Check sheet for the drawn part. Datum: minimum x, y, z corner. Units: mm. A direction names the side the tool comes from. Round coordinates to 2 decimals unless told otherwise and drop trailing zeros. Write each loop counter-clockwise with the first axis right and the second up, starting at its lowest first coordinate (ties: lowest second). Pieces come first, ordered by that corner, then holes.
Item 1: Cross-section at D-D on x = 2.5. Enter the section's corners in (y, z).
Item 2: Release check for a two-part mould opening along Z. For the marked faces 3, 4 and 5 record: +Z half, -Z half, draft (parallel to the pull), parting line (faces both ways), or undercut.
Item 3: Cross-section at C-C on x = 17.25. Enter the section's corners in (y, z).
Item 4: Tool access check on the marked faces 1 and 2. Record the directions out of +Z, -Z, +X, -X, +Y, -Y that give a thin tool (end or side, any length) a straight path to the whole face; none if there is none.
Item 5: Material ranges on line 1 (X direction, y = 0.95, z = 2.9); line 2 (X direction, y = 1.2, z = 4.15); line 3 (Z direction, x = 14.5, y = 0.85), recorded low to high.
Item 6: Cross-section at B-B on y = 1.25. Enter the section's corners in (x, z).
Item 7: Cross-section at A-A on z = 3. Enter the section's corners in (x, y), plus the area to 3 significant figures.
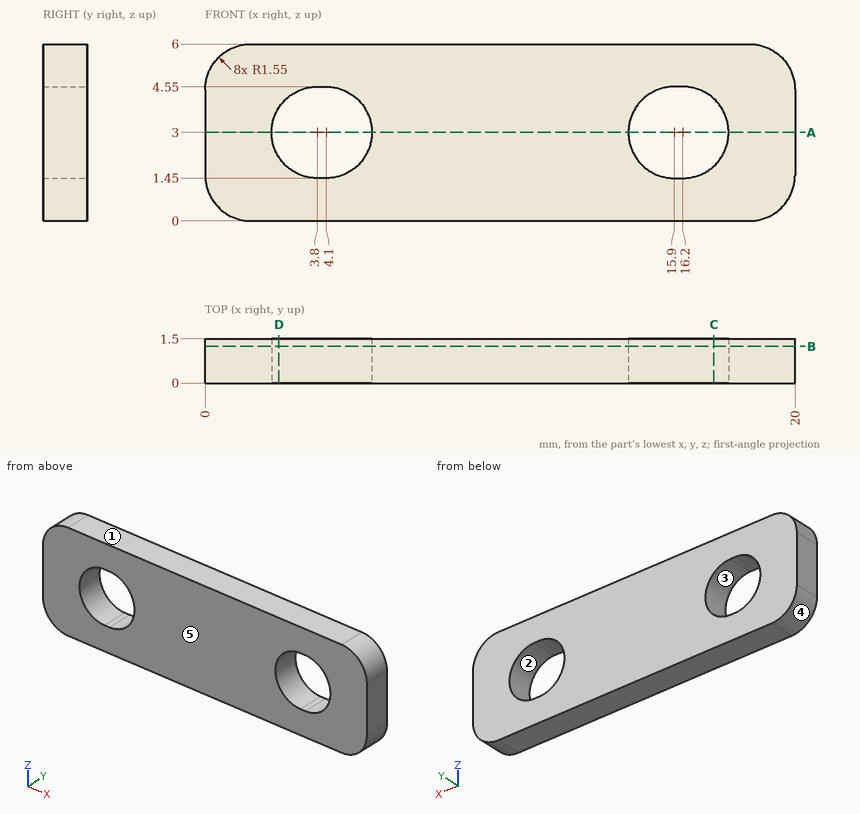
Response values:
1. outline: (0, 0) - (1.5, 0) - (1.5, 2.16) - (0, 2.16) - close; (0, 3.84) - (1.5, 3.84) - (1.5, 6) - (0, 6) - close
2. face 3: undercut
2. face 4: -Z half
2. face 5: draft
3. outline: (0, 0) - (1.5, 0) - (1.5, 1.86) - (0, 1.86) - close; (0, 4.14) - (1.5, 4.14) - (1.5, 6) - (0, 6) - close
4. face 1: +Z, +X, -X, +Y, -Y
4. face 2: +Y, -Y
5. line 1: x = 0 to 2.25, 5.65 to 14.35, 17.75 to 20
5. line 2: x = 0 to 2.76, 5.14 to 14.86, 17.24 to 20
5. line 3: z = 0 to 2.33, 3.67 to 6
6. outline: (0, 1.55) arc R1.55 ccw to (1.55, 0) - (18.45, 0) arc R1.55 ccw to (20, 1.55) - (20, 4.45) arc R1.55 ccw to (18.45, 6) - (1.55, 6) arc R1.55 ccw to (0, 4.45) - close; hole (3.8, 1.45) - (4.1, 1.45) arc R1.55 ccw to (4.1, 4.55) - (3.8, 4.55) arc R1.55 ccw to start; hole (15.9, 1.45) - (16.2, 1.45) arc R1.55 ccw to (16.2, 4.55) - (15.9, 4.55) arc R1.55 ccw to start
7. outline: (0, 0) - (2.25, 0) - (2.25, 1.5) - (0, 1.5) - close; (5.65, 0) - (14.35, 0) - (14.35, 1.5) - (5.65, 1.5) - close; (17.75, 0) - (20, 0) - (20, 1.5) - (17.75, 1.5) - close
7. area: 19.8 mm2
